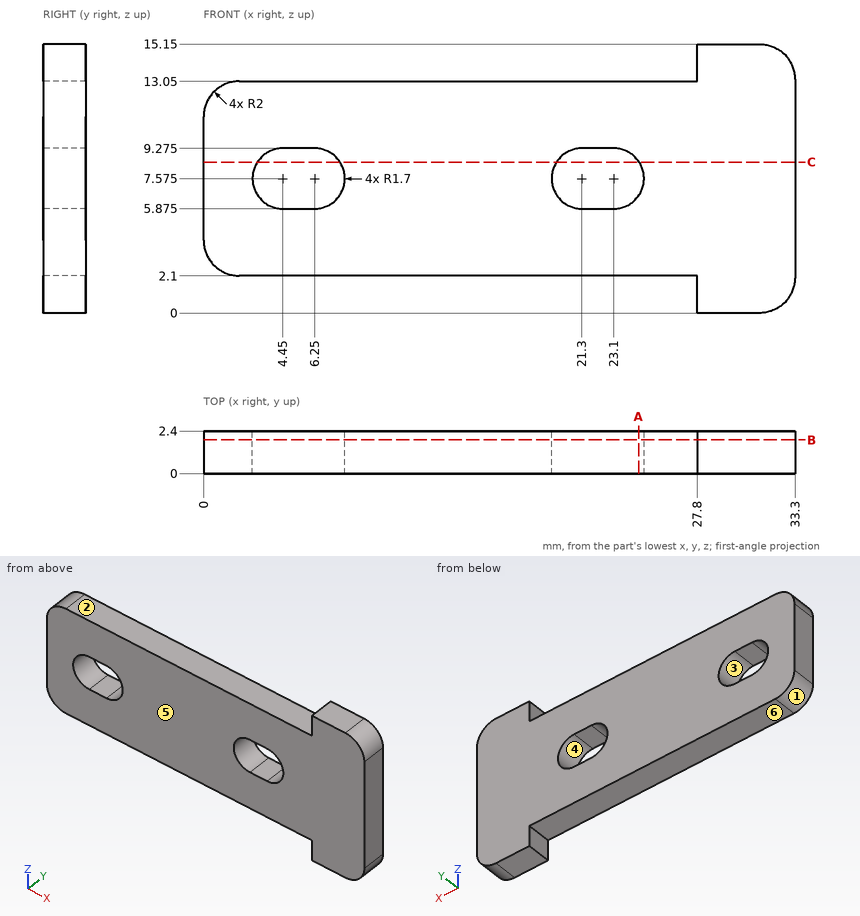
Here's the drawing with two shaded views (mm, measured from the low corner). I have some questions. A direction names the side the tool comes from. Give positions to 0.01 mm unless a question says otherwise; leave off trailing zeros. Write each loop counter-clockwise with the first axis right and the second up, starting at its lowest first coordinate (ties: lowest second). Pieces come first, ordered by that corner, then holes. Notation, with made-up numbers: (71, -12) -> (114, -12) arc R19 cw to (114, -2) -> close; hole circle Ø6 at (-23.75, 3). An arc over 180 degrees is marked (long way). One line per item, written item: value.
Q1. For P1, Ø0.5, axis at x = 22.5, y = 0.5, coming from the -Z side; P2, Ø0.7, axis at x = 16, y = 1, coming from the +Z side, each with a flat end and sliding along its axis, tell me the tip position at first contact or that it passes through.
Results found:
P1: stops at z = 2.1
P2: stops at z = 13.05
Q2. Imagine slicing it at A-A on x = 24.5. Please give me the cut outline in (y, z), and give its area (3 significant figures).
Results found:
outline: (0, 2.1) -> (2.4, 2.1) -> (2.4, 6.61) -> (0, 6.61) -> close; (0, 8.54) -> (2.4, 8.54) -> (2.4, 13.05) -> (0, 13.05) -> close
area: 21.7 mm^2
Q3. Please list where these lines run through material, in increasing order: line 1 (Z direction, x = 21.5, y = 1.3) (3 decimals); line 2 (X direction, y = 0.35, z = 8.75); line 3 (Z direction, x = 2, y = 0.1). Write a range as [from, to].
Results found:
line 1: z = [2.1, 5.875], [9.275, 13.05]
line 2: x = [0, 3.22], [7.48, 20.07], [24.33, 33.3]
line 3: z = [2.1, 13.05]
Q4. Imagine slicing it at B-B on y = 1.9. Please give me the cut outline in (x, z) (3 decimals), and give its area (3 significant figures).
Results found:
outline: (0, 4.1) arc R2 ccw to (2, 2.1) -> (27.8, 2.1) -> (27.8, 0) -> (31.3, 0) arc R2 ccw to (33.3, 2) -> (33.3, 13.15) arc R2 ccw to (31.3, 15.15) -> (27.8, 15.15) -> (27.8, 13.05) -> (2, 13.05) arc R2 ccw to (0, 11.05) -> close; hole (4.45, 5.875) -> (6.25, 5.875) arc R1.7 ccw to (6.25, 9.275) -> (4.45, 9.275) arc R1.7 ccw to start; hole (21.3, 5.875) -> (23.1, 5.875) arc R1.7 ccw to (23.1, 9.275) -> (21.3, 9.275) arc R1.7 ccw to start
area: 354 mm^2
Q5. Imagine slicing it at C-C on z = 8.5. Please give me the cut outline in (x, y), and give its area (3 significant figures).
Results found:
outline: (0, 0) -> (3.02, 0) -> (3.02, 2.4) -> (0, 2.4) -> close; (7.68, 0) -> (19.87, 0) -> (19.87, 2.4) -> (7.68, 2.4) -> close; (24.53, 0) -> (33.3, 0) -> (33.3, 2.4) -> (24.53, 2.4) -> close
area: 57.6 mm^2
Q6. We'd pull the mould along X, two halves only. Please class the marked faces 1, 2 and 3: +X half, -X half, draft (parallel to the pull), parting line (faces both ways), or undercut.
Results found:
face 1: -X half
face 2: draft
face 3: undercut
Q7. Which directions (+Z, -Z, +X, -X, +Y, -Y) give clear straight access to the entire face, cutting with the end or side of a thin tool? Please do the marked faces 4, 5 and 6.
Results found:
face 4: +Y, -Y
face 5: +Z, -Z, +X, -X, -Y
face 6: -Z, -X, +Y, -Y
